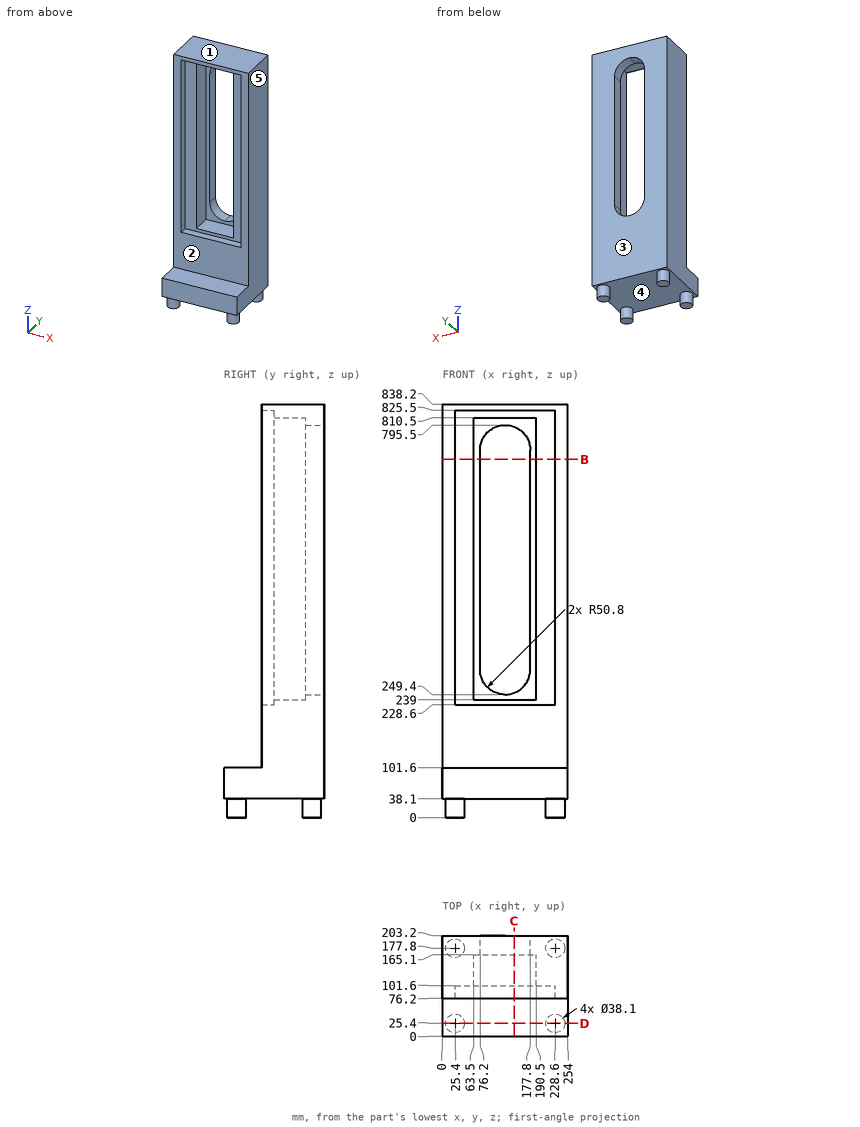
Geometry: see drawing. Coordinates: mm, zero at the bounding-box minimum. A direction names the side the tool comes from. Coordinates: 2 decimals unless noted, no trailing zeros. Order: outer loops, then holes, each group sorted by start corner. A loop starts at its lowest first (then second) coordinate and runs counter-clockwise, first axis right, second up. Notation, with made-up numbers: M 15.25,2.5 L 62.25,2.5 A10 ccw 62.25,16.5 Z; hole C -6.75,11.25 d5. An arc over 180 degrees is marked long. Answer in a Markdown table with one row per item. Add a question column.
Q1. Reachability of the marked faces 1 and 2 from +Z, -Z, +X, -X, +Y, -Y: full face, straight path, thin tool, end or side. Return the list, or none.
Q2. Contact query for a flat-ended pin moving along its axis: P1, Ø1, axis at x = 55, y = 161.5, coming from the -Z side. Output: stop coordinate, or through.
Q3. Mould query, pull axis Y, two halves, no side actions, for the marked faces 3, 4 and 5. Classes: released by +Y, released by -Y, zero draft, split by the parting line, or undercut.
Q4. Line query: L1, parallel to X at y = 187.5, z = 713; L2, parallel to X at y = 101.5, z = 471; L3, parallel to Z at x = 167.5, y = 158.5. Output: solid intervals per line, ascending.
Q5. Section query C-C on x = 145. Return the cut outline in (y, z).
Q6. Section query D-D on y = 25.4. Return the cut outline in (x, z).
Q7. Section query B-B on z = 726. Return the cut outline in (x, y), and give its area (3 significant figures).
Completed:
| question | item | result |
|---|---|---|
| 1 | face 1 | +Z, +X, -X, +Y, -Y |
| 1 | face 2 | +Z, +X, -X, -Y |
| 2 | P1 | stops at z = 38.1 |
| 3 | face 3 | released by +Y |
| 3 | face 4 | undercut |
| 3 | face 5 | zero draft |
| 4 | L1 | x = 0 to 76.2, 177.8 to 254 |
| 4 | L2 | x = 0 to 25.4, 228.6 to 254 |
| 4 | L3 | z = 38.1 to 239, 810.5 to 838.2 |
| 5 | outline | M 0,38.1 L 203.2,38.1 L 203.2,252.7 L 165.1,252.7 L 165.1,239 L 101.6,239 L 101.6,228.6 L 76.2,228.6 L 76.2,101.6 L 0,101.6 Z; M 76.2,825.5 L 101.6,825.5 L 101.6,810.5 L 165.1,810.5 L 165.1,792.2 L 203.2,792.2 L 203.2,838.2 L 76.2,838.2 Z |
| 6 | outline | M 0,38.1 L 6.35,38.1 L 6.35,0 L 44.45,0 L 44.45,38.1 L 209.55,38.1 L 209.55,0 L 247.65,0 L 247.65,38.1 L 254,38.1 L 254,101.6 L 0,101.6 Z |
| 7 | outline | M 0,76.2 L 25.4,76.2 L 25.4,101.6 L 63.5,101.6 L 63.5,165.1 L 76.2,165.1 L 76.2,203.2 L 0,203.2 Z; M 177.8,165.1 L 190.5,165.1 L 190.5,101.6 L 228.6,101.6 L 228.6,76.2 L 254,76.2 L 254,203.2 L 177.8,203.2 Z |
| 7 | area | 15,200 mm2 |
